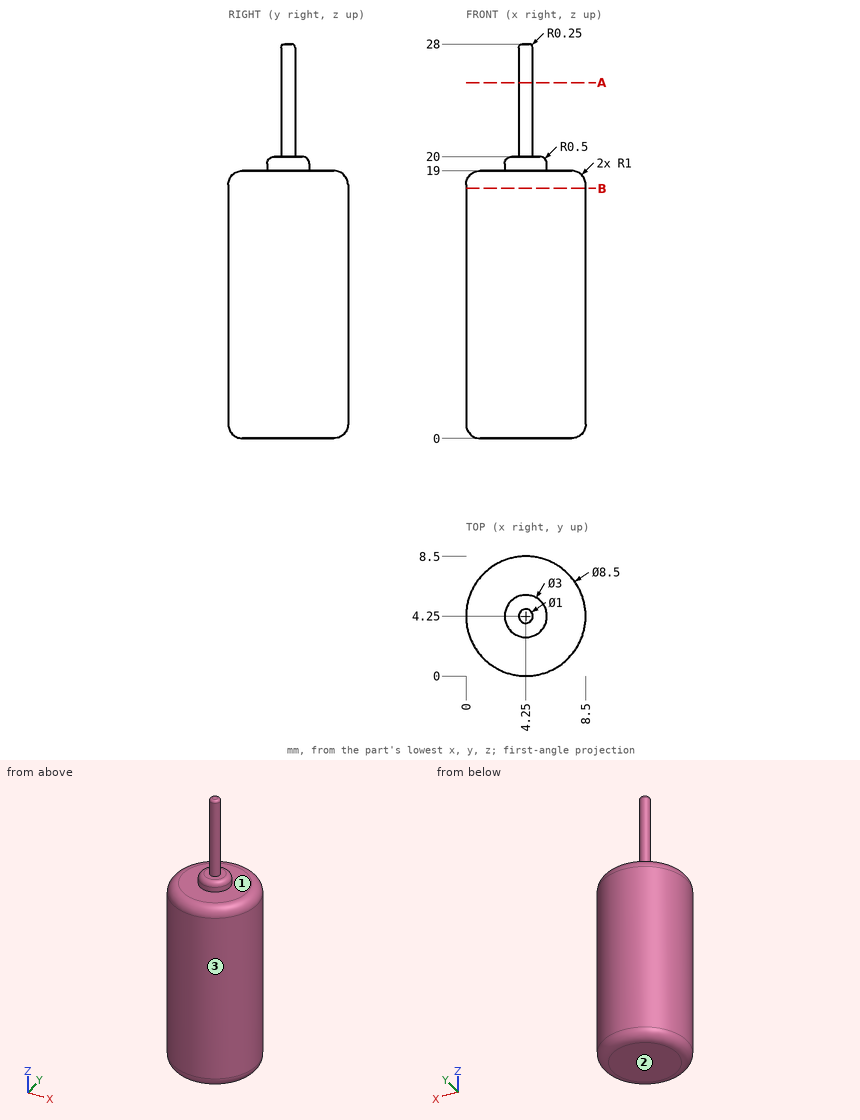
Geometry: see drawing. Coordinates: mm, zero at the bounding-box minimum. Coordinates: 2 decimals unless noted, no trailing zeros. Loops run counter-clockwise (first coordinate to the right, second up) from the corner with the lowest first, then second, coordinate; pieces in that order, holes last.
(1) First-contact query: pin 1 Ø1 at (x, y) = (6, 5.5) entering from +Z; pin 2 Ø4 at (x, z) = (1.5, 12) entering from -Y; pin 3 Ø3 at (y, z) = (6.5, 17) entering from +X. Flat tips, straight axial feed; report the tip coordinate or a pass-through.
(2) Pull-direction query (Z, two-part tool) for the marked faces 1, 2 and 3; classes: released by +Z, released by -Z, zero draft, split by the parting line, or undercut.
(3) Section B-B on z = 17.75. Return the cut outline in (x, y), then the cut area to 3 significant figures.
(4) Material intervals for probe 1 along Z at (x, y) = (1.5, 3); probe 2 along Y at (x, z) = (4, 3); probe 3 along Y at (x, z) = (8, 2.5), sorted ascending.
(5) Section A-A on z = 25.25. Return the cut outline in (x, y), then the cut area to 3 significant figures.
Data:
1. pin 1: stops at z = 19
1. pin 2: stops at y = 0.07
1. pin 3: stops at x = 8.43
2. face 1: released by +Z
2. face 2: released by -Z
2. face 3: zero draft
3. outline: circle Ø8.5 at (4.25, 4.25)
3. area: 56.7 mm2
4. probe 1: z = 0 to 19
4. probe 2: y = 0.01 to 8.49
4. probe 3: y = 2.25 to 6.25
5. outline: circle Ø1 at (4.25, 4.25)
5. area: 0.785 mm2
